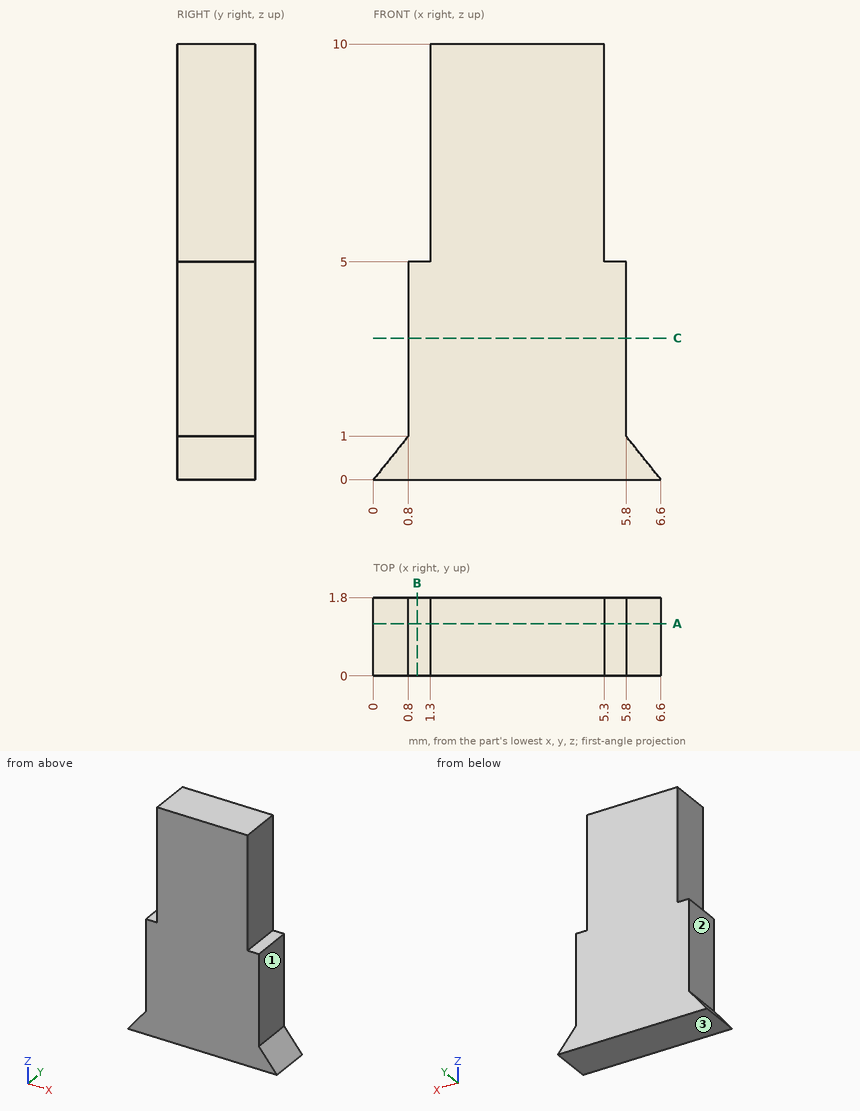
Verification items for this drawing (mm, ordinates from the low corner). A direction names the side the tool comes from. Coordinates: 2 decimals unless noted, no trailing zeros. Order: outer loops, then holes, each group sorted by start corner. A loop starts at its lowest first (then second) coordinate and runs counter-clockwise, first axis right, second up. Notation, with made-up numbers: (36.25, 53.25) - (80.25, 53.25) arc R13 cw to (80.25, 75.25) - close; hole circle Ø6 at (-15.5, 35). An arc over 180 degrees is marked (long way). Answer in a Markdown table with one row per item. Add a question column.
1. Gauge pin test, flat end, axial feed: pin 1 Ø0.5 at (y, z) = (1, 4) entering from +X. Record the tip position at first contact, or that the pin passes through.
2. Material ranges on L1, parallel to X at y = 1.2, z = 8.5; L2, parallel to Z at x = 1.25, y = 1.55; L3, parallel to X at y = 0.7, z = 3.5, recorded low to high. Write a range as [from, to].
3. Section check A-A (y = 1.2). Enter the section's corners in (x, z).
4. Access from +Z, -Z, +X, -X, +Y, -Y to the whole of each face (thin tool, end or side, straight path). Record for the marked faces 1, 2 and 3.
5. Section check B-B (x = 1). Enter the section's corners in (y, z), plus the area to 3 significant figures.
6. Section check C-C (z = 3.25). Enter the section's corners in (x, y).
Data:
| question | item | result |
|---|---|---|
| 1 | pin 1 | stops at x = 5.8 |
| 2 | L1 | x = [1.3, 5.3] |
| 2 | L2 | z = [0, 5] |
| 2 | L3 | x = [0.8, 5.8] |
| 3 | outline | (0, 0) - (6.6, 0) - (5.8, 1) - (5.8, 5) - (5.3, 5) - (5.3, 10) - (1.3, 10) - (1.3, 5) - (0.8, 5) - (0.8, 1) - close |
| 4 | face 1 | +Z, +X, +Y, -Y |
| 4 | face 2 | +Z, -X, +Y, -Y |
| 4 | face 3 | -Z, +X, -X, +Y, -Y |
| 5 | outline | (0, 0) - (1.8, 0) - (1.8, 5) - (0, 5) - close |
| 5 | area | 9.00 mm² |
| 6 | outline | (0.8, 0) - (5.8, 0) - (5.8, 1.8) - (0.8, 1.8) - close |
